```python
from build123d import *

# Parameters (mm, degrees)
BOSS_EXTRUDE1_DEPTH = 1.524


with BuildPart() as part:
    # Sketch1 → Boss-Extrude1 (new body)
    with BuildSketch(Plane.XY):
        with BuildLine():
            Line((79.357173925, 0), (79.357173925, -1.524))
            Line((79.357173925, -1.524), (27.997218561, -1.524))
            ThreePointArc((27.997218561, -1.524), (28.839303716, -3.893478834), (30.585272442, -5.703211014))
            ThreePointArc((30.585272442, -5.703211014), (35.473881568, -10.546204028), (37.343248984, -17.168782529))
            ThreePointArc((37.343248984, -17.168782529), (37.371863233, -17.198154529), (37.400490384, -17.227513955))
            ThreePointArc((37.400490384, -17.227513955), (84.54475886, -25.491518967), (125.974625666, -1.524))
            Line((125.974625666, -1.524), (126.331576391, -0.762))
            Line((126.331576391, -0.762), (125.974625666, 0))
            ThreePointArc((125.974625666, 0), (84.54475886, 23.967518967), (37.400490384, 15.703513955))
            ThreePointArc((37.400490384, 15.703513955), (37.371863233, 15.674154529), (37.343248984, 15.644782529))
            ThreePointArc((37.343248984, 15.644782529), (35.473881568, 9.022204028), (30.585272442, 4.179211014))
            ThreePointArc((30.585272442, 4.179211014), (28.839303716, 2.369478834), (27.997218561, 0))
            Line((27.997218561, 0), (79.357173925, 0))
        make_face()
    extrude(amount=BOSS_EXTRUDE1_DEPTH)


solid = part.part
```
Verification items for the finished model (mm, model axes). Give positions to 0.01 mm unless a question says otherwise; leave off trailing zeros. Loops run counter-clockwise (first coordinate to the right, second up) from the corner with the lowest first, then second, coordinate; pieces in that order, holes last.
1. Section check D-D, the plane x = 116.5. Enter the section's corners in (y, z).
2. Mould release check, pull along Z, two halves, no side actions. Record for faces 1 (the flat face through (76, 5, 1.524)), 2 (the cylindrical face through (28.86, 2.4, 0.75)), 3 (the flat face through (76, 5, 0)): released by +Z, released by -Z, zero draft, split by the parting line, or undercut.
3. Go/stop test with a flat-tipped pin: pin 1 Ø0.5 at (x, z) = (66.5, 1) entering from -Y. Record where the tip stops, or that it passes through.
4. Section check B-B, the plane z = 0.9. Enter the section's corners in (x, y), then the cut area to 3 significant figures.
5. Thickness scan on line 1 (Y direction, x = 42.5, z = 0.75); line 2 (Y direction, x = 57.5, z = 0.3); line 3 (X direction, y = -20.5, z = 1.3). Record the ranges inside material, lowest first.
6. Section check A-A, the plane x = 53.5. Enter the section's corners in (y, z).
7. Section check C-C, the plane y = 14. Enter the section's corners in (x, z), then the cut area to 3 significant figures.
Geometry says:
1. outline: (-10.86, 0) - (9.34, 0) - (9.34, 1.52) - (-10.86, 1.52) - close
2. face 1: released by +Z
2. face 2: zero draft
2. face 3: released by -Z
3. pin 1: stops at y = -26.34
4. outline: (28, -1.52) arc R5.95 ccw to (30.59, -5.7) arc R13.51 cw to (37.34, -17.17) arc R93.33 ccw to (37.4, -17.23) arc R69.98 ccw to (125.97, -1.52) - (126.33, -0.76) - (125.97, 0) arc R69.98 ccw to (37.4, 15.7) arc R93.33 ccw to (37.34, 15.64) arc R13.51 cw to (30.59, 4.18) arc R5.95 ccw to (28, 0) - (79.36, 0) - (79.36, -1.52) - close
4. area: 3,590 mm2
5. line 1: y = -19.89 to -1.52, 0 to 18.37
5. line 2: y = -24.98 to -1.52, 0 to 23.45
5. line 3: x = 43.83 to 100.83
6. outline: (-23.99, 0) - (-1.52, 0) - (-1.52, 1.52) - (-23.99, 1.52) - close; (0, 0) - (22.46, 0) - (22.46, 1.52) - (0, 1.52) - close
7. outline: (37.21, 0) - (110.06, 0) - (110.06, 1.52) - (37.21, 1.52) - close
7. area: 111 mm2
